The listing builds one solid part. Answer for the finished solid, in the listing's coordinates (mm). Round coordinates to 2 decimals unless told otherwise and drop trailing zeros. Write each loop counter-clockwise with the first axis right and the second up, starting at its lowest first coordinate (ties: lowest second). Pieces come first, ordered by that corner, then holes. Notation, with made-up numbers: M -2.5,-23 L 24.5,-23 A16 ccw 24.5,6 Z; hole C -29,-21.5 d5. An arc over 180 degrees is marked long. Answer as CSV lines item,"result". Start each with the question number.
from build123d import *

# Parameters (mm, degrees)
EXTRUDE_1_DEPTH     = 5
SKETCH_2_R          = 3
CUT_EXTRUDE_1_DEPTH = 5
CUT_EXTRUDE_2_DEPTH = 10
FILLET_2_R          = 10


with BuildPart() as part:
    # 스케치1 → 보스-돌출1 (new body)
    with BuildSketch(Plane(origin=(0, 0, 0), x_dir=(0, 0, -1), z_dir=(1, 0, 0))):
        Polygon((0, 150), (100, 50), (100, 0), (0, 0), align=None)
    extrude(amount=EXTRUDE_1_DEPTH)

    # 스케치2 → 컷-돌출1 (cut)
    with BuildSketch(Plane(origin=(5, 0, 0), x_dir=(0, 0, -1), z_dir=(1, 0, 0))):
        with Locations((45, 95)):
            Circle(SKETCH_2_R)
    extrude(amount=-CUT_EXTRUDE_1_DEPTH, mode=Mode.SUBTRACT)

    # 스케치3 → 컷-돌출2 (cut)
    with BuildSketch(Plane(origin=(5, 0, 0), x_dir=(0, 0, -1), z_dir=(1, 0, 0))):
        Polygon((35, 115), (0, 80), (0, 150), align=None)
    extrude(amount=-CUT_EXTRUDE_2_DEPTH, mode=Mode.SUBTRACT)

    # 필렛2
    fillet_2_edges = [part.edges().sort_by_distance(p)[0] for p in [
        (2.5, 115, -35),
        (2.5, 80, 0),
        (2.5, 50, -100),
    ]]
    fillet(fillet_2_edges, radius=FILLET_2_R)


solid = part.part
Q1. Straight lines are drawn through the part: L1, parallel to Y at x = 3.35, z = -45; L2, parallel to Y at x = 3.75, z = -38; L3, parallel to Y at x = 0.9, z = -77.5. For each, find the intervals that lie inside material, in ascending order.
Q2. Find section C-C (y = 95). Determine the outline of the cut face in (x, z), plus the area to 3 significant figures.
Q3. Find section D-D (z = -92). Determine the outline of the cut face in (x, y).
Q4. Find section B-B (x = 2.9). Determine the outline of the cut face in (y, z), plus the area to 3 significant figures.
Q5. This flat-tipped pin is pushed along its axis until it touches: P1, Ø3.5, axis at y = 95, z = -45, coming from the -X side. Where does it stop, or does it pass through?
Q6. Find section A-A (z = -45). Determine the outline of the cut face in (x, y), plus the area to 3 significant figures.
Q7. The mould has two halves that part along Z. Classify faces 1 (the face through (2.54, 92.07, -44.35)), 2 (the face through (2, 81, -69)), 3 (the face through (2, 0, -51)), 4 (the face through (2.465, 110.857, -35.11)): +Z half, -Z half, draft (parallel to the pull), parting line (faces both ways), or undercut.
Reported:
1,L1,"y = 0 to 92, 98 to 105"
1,L2,"y = 0 to 110.4"
1,L3,"y = 0 to 72.5"
2,outline,"M 0,-55 L 5,-55 L 5,-48 L 0,-48 Z; M 0,-42 L 5,-42 L 5,-15 L 0,-15 Z"
2,area,"170 mm2"
3,outline,"M 0,0 L 5,0 L 5,58 L 0,58 Z"
4,outline,"M 0,-100 L 45.86,-100 A10 ccw 52.93,-97.07 L 107.93,-42.07 A10 ccw 107.93,-27.93 L 82.93,-2.93 A10 ccw 75.86,0 L 0,0 Z; hole C 95,-45 d6"
4,area,"8,720 mm2"
5,P1,"passes through"
6,outline,"M 0,0 L 5,0 L 5,92 L 0,92 Z; M 0,98 L 5,98 L 5,105 L 0,105 Z"
6,area,"495 mm2"
7,face 1,"undercut"
7,face 2,"-Z half"
7,face 3,"draft"
7,face 4,"parting line"
